Could you check a few things on this model? Use its own coordinates, in mm. A direction names the side the tool comes from. Give positions to 0.01 mm unless a question says otherwise; leave off trailing zeros. Write each loop counter-clockwise with the first axis right and the second up, starting at its lowest first coordinate (ties: lowest second). Pieces come first, ordered by that corner, then holes. Notation, with made-up numbers: (19.5, -39.5) -> (74.5, -39.5) arc R8 ccw to (74.5, -30.5) -> close; hole circle Ø7 at (65.25, 13.5). An arc over 180 degrees is marked (long way). One line per question, with ' | ' between items.
from build123d import *

# Parameters (mm, degrees)
SKETCH1_R           = 6
BOSS_EXTRUDE1_DEPTH = 4
SKETCH2_R           = 4
BOSS_EXTRUDE2_DEPTH = 29
SKETCH3_R           = 2.5
BOSS_EXTRUDE3_DEPTH = 17
CHAMFER1_SIZE       = 0.5
CHAMFER2_SIZE       = 1
SKETCH4_R           = 2.5
CUT_EXTRUDE1_DEPTH  = 1
FILLET1_R           = 0.5


with BuildPart() as part:
    # Sketch1 → Boss-Extrude1 (new body)
    with BuildSketch(Plane(origin=(0, 0, 0), x_dir=(0, 0, -1), z_dir=(1, 0, 0))):
        Circle(SKETCH1_R)
    extrude(amount=BOSS_EXTRUDE1_DEPTH)

    # Sketch2 → Boss-Extrude2 (add)
    with BuildSketch(Plane(origin=(4, 0, 0), x_dir=(0, 0, -1), z_dir=(1, 0, 0))):
        Circle(SKETCH2_R)
    extrude(amount=BOSS_EXTRUDE2_DEPTH)

    # Sketch3 → Boss-Extrude3 (add)
    with BuildSketch(Plane(origin=(33, 0, 0), x_dir=(0, 0, -1), z_dir=(1, 0, 0))):
        Circle(SKETCH3_R)
    extrude(amount=BOSS_EXTRUDE3_DEPTH)

    # Chamfer1
    chamfer1_edges = [part.edges().sort_by_distance(p)[0] for p in [
        (50, 0, 2.5),
    ]]
    chamfer(chamfer1_edges, length=CHAMFER1_SIZE)

    # Chamfer2
    chamfer2_edges = [part.edges().sort_by_distance(p)[0] for p in [
        (0, 0, 6),
    ]]
    chamfer(chamfer2_edges, length=CHAMFER2_SIZE)

    # Sketch4 → Cut-Extrude1 (cut)
    with BuildSketch(Plane.ZY):
        Circle(SKETCH4_R)
    extrude(amount=-CUT_EXTRUDE1_DEPTH, mode=Mode.SUBTRACT)

    # Fillet1
    fillet1_edges = [part.edges().sort_by_distance(p)[0] for p in [
        (0, 0, -2.5),
    ]]
    fillet(fillet1_edges, radius=FILLET1_R)


solid = part.part
Q1. Imagine slicing it at A-A on z = 0. Please give me the cut outline in (x, y), and give its area (3 significant figures).
Answer below:
outline: (0, -5) -> (1, -6) -> (4, -6) -> (4, -4) -> (33, -4) -> (33, -2.5) -> (49.5, -2.5) -> (50, -2) -> (50, 2) -> (49.5, 2.5) -> (33, 2.5) -> (33, 4) -> (4, 4) -> (4, 6) -> (1, 6) -> (0, 5) -> (0, 3) arc R0.5 ccw to (0.5, 2.5) -> (1, 2.5) -> (1, -2.5) -> (0.5, -2.5) arc R0.5 ccw to (0, -3) -> close | area: 359 mm^2
Q2. Imagine slicing it at D-D on x = 39.5. Please give me the cut outline in (y, z).
Answer below:
outline: circle Ø5 at (0, 0)
Q3. On a 3-axis mill with a long thin cutter (end or side, diameter ignored), from which of +Z, -Z, +X, -X, +Y, -Y can I reach the whole of each face in a straight line? I mean faces 4 (the cylindrical face through (18.297, -3.905, 0.867)), 5 (the flat face through (50, 0, 0)), 6 (the flat face through (1, 0, 0)). Say none if no direction works.
Answer below:
face 4: +X | face 5: +Z, -Z, +X, +Y, -Y | face 6: -X
Q4. Will these pins go through, and if not, where does the flat tip stop? pin 1 (1 mm diameter, centred on x = 7, z = -0.5, fed in from +Y); pin 2 (1.5 mm diameter, centred on y = 0.5, z = -0.5, fed in from -X); pin 3 (1 mm diameter, centred on x = 32.5, y = -2, fed in from +Z).
Answer below:
pin 1: stops at y = 4 | pin 2: stops at x = 1 | pin 3: stops at z = 3.71
Q5. Imagine slicing it at C-C on x = 5. Please give me the cut outline in (y, z).
Answer below:
outline: circle Ø8 at (0, 0)
Q6. If I drill on line 1 along X through (y, z) = (-2.25, -3); line 2 along X through (y, z) = (-0.5, -1.25); line 3 along Y through (x, z) = (45, 1.5), over which ranges is the centre line in solid material (lowest first)?
Answer below:
line 1: x = 0 to 33 | line 2: x = 1 to 50 | line 3: y = -2 to 2
Q7. If we mould it in two halves opening along Y, with no side actions, what happens to faces 1 (the cylindrical face through (41.13, -2.44, 0.54)), 2 (the flat face through (0, -3.3, 0.1)), 3 (the cylindrical face through (0.75, -2.44, -0.54))? For each: +Y half, -Y half, draft (parallel to the pull), parting line (faces both ways), or undercut.
Answer below:
face 1: parting line | face 2: draft | face 3: undercut
